Input: part model. Units: mm. Frame: model coordinates. A direction names the side the tool comes from. Round coordinates to 2 decimals unless told otherwise and drop trailing zeros. Loops run counter-clockwise (first coordinate to the right, second up) from the corner with the lowest first, then second, coordinate; pieces in that order, holes last. Notation, with made-up numbers: (59, 35) -> (94, 35) arc R27 cw to (94, 59) -> close; hole circle Ø1 at (75, 17.25). An arc over 180 degrees is marked (long way). Answer as a JSON object with one key per item and string values. Group by question number.
Item 1: Pin query (flat end, axial travel): pin 1 (1.5 mm diameter, centred on x = 57, y = 54, fed in from -Z). Return the tip coordinate at first contact, or that it passes through.
Item 2: Draft query along Y for faces 5 (the flat face through (1, 154, -26)), 6 (the flat face through (-100, 76, 1)), 7 (the flat face through (-93, 78, 1)), 8 (the flat face through (-1, 78, -93)). Return one class per face: released by +Y, released by -Y, zero draft, split by the parting line, or undercut.
Item 3: Section query A-A on x = -15. Return loops of the section in (y, z), and give its area (3 significant figures).
Item 4: Set-up query: faces 1 (the flat face through (1, 76, 100)), 2 (the flat face through (-1, 76, -100)), 3 (the cylindrical face through (23.846, 0.986, -7.509)), 4 (the flat face through (-22, 2, -22)). Return all of +Z, -Z, +X, -X, +Y, -Y with unobstructed straight access to the full face (end or side cutting, diameter ignored); none if empty.
Item 5: Section query B-B on z = 0. Return loops of the section in (x, y), and give its area (3 significant figures).
Item 6: Section query C-C on x = -90. Return loops of the section in (y, z), and give its area (3 significant figures).
Item 7: Material intervals for line 1 (Y direction, x = -76, z = 6); line 2 (X direction, y = 52.5, z = 100.5); line 3 (Z direction, x = -67, y = 19.5), sorted ascending. Write a range as [from, to].
Item 8: Section query D-D on y = 32.5. Return loops of the section in (x, z).
from build123d import *

# Parameters (mm, degrees)
SKETCH1_R           = 25
BOSS_EXTRUDE1_DEPTH = 154
SKETCH2_W           = 186
SKETCH2_H           = 186
CUT_EXTRUDE1_DEPTH  = 150


with BuildPart() as part:
    # Sketch1 → Boss-Extrude1 (new body)
    with BuildSketch(Plane(origin=(0, 0, 0), x_dir=(1, 0, 0), z_dir=(0, 1, 0))):
        with BuildLine():
            Line((-80, 100), (80, 100))
            ThreePointArc((80, 100), (90, 110), (100, 100))
            Line((100, 100), (100, -100))
            ThreePointArc((100, -100), (90, -110), (80, -100))
            Line((80, -100), (-80, -100))
            ThreePointArc((-80, -100), (-90, -110), (-100, -100))
            Line((-100, -100), (-100, 100))
            ThreePointArc((-100, 100), (-90, 110), (-80, 100))
        make_face()
        Circle(SKETCH1_R, mode=Mode.SUBTRACT)
    extrude(amount=BOSS_EXTRUDE1_DEPTH)

    # Sketch2 → Cut-Extrude1 (cut)
    with BuildSketch(Plane(origin=(0, 152, 0), x_dir=(1, 0, 0), z_dir=(0, 1, 0))):
        Rectangle(SKETCH2_W, SKETCH2_H)
    extrude(amount=-CUT_EXTRUDE1_DEPTH, mode=Mode.SUBTRACT)


solid = part.part
Solved:
{
 "1": {"pin 1": "z = -100"},
 "2": {"face 5": "released by +Y", "face 6": "zero draft", "face 7": "undercut", "face 8": "undercut"},
 "3": {"outline": "(0, -100) -> (154, -100) -> (154, -20) -> (152, -20) -> (152, -93) -> (2, -93) -> (2, -20) -> (0, -20) -> close; (0, 20) -> (2, 20) -> (2, 93) -> (152, 93) -> (152, 20) -> (154, 20) -> (154, 100) -> (0, 100) -> close", "area": "2,740 mm²"},
 "4": {"face 1": "+Z, +Y, -Y", "face 2": "-Z, +Y, -Y", "face 3": "+Y, -Y", "face 4": "none"},
 "5": {"outline": "(-100, 0) -> (-25, 0) -> (-25, 2) -> (-93, 2) -> (-93, 152) -> (-25, 152) -> (-25, 154) -> (-100, 154) -> close; (25, 0) -> (100, 0) -> (100, 154) -> (25, 154) -> (25, 152) -> (93, 152) -> (93, 2) -> (25, 2) -> close", "area": "2,700 mm²"},
 "6": {"outline": "(0, -110) -> (154, -110) -> (154, 110) -> (0, 110) -> close; hole (2, -93) -> (152, -93) -> (152, 93) -> (2, 93) -> close", "area": "5,980 mm²"},
 "7": {"line 1": "[0, 2], [152, 154]", "line 2": "[-99.99, -80.01], [80.01, 99.99]", "line 3": "[-100, -93], [93, 100]"},
 "8": {"outline": "(-100, -100) arc R10 ccw to (-80, -100) -> (80, -100) arc R10 ccw to (100, -100) -> (100, 100) arc R10 ccw to (80, 100) -> (-80, 100) arc R10 ccw to (-100, 100) -> close; hole (-93, -93) -> (93, -93) -> (93, 93) -> (-93, 93) -> close"}
}
